```python
from build123d import *

# Parameters (mm, degrees)
SKETCH_1_R          = 9
EXTRUDE_1_DEPTH     = 65
SKETCH_2_R          = 6.5
SKETCH_2_R_2        = 5
CUT_EXTRUDE_1_DEPTH = 2
SKETCH_3_R          = 7.5
CUT_EXTRUDE_2_DEPTH = 0.25
CUT_EXTRUDE_START   = 1
SKETCH_4_R          = 6.75
SKETCH_4_R_2        = 5
CUT_EXTRUDE_3_DEPTH = 1
FILLET_1_R          = 1.5
FILLET_2_R          = 0.5
FILLET_3_R          = 0.5


with BuildPart() as part:
    # 草图1 → 凸台-拉伸1 (new body)
    with BuildSketch(Plane(origin=(0, 0, 0), x_dir=(1, 0, 0), z_dir=(0, 1, 0))):
        with Locations(Location((0, 0, 0), (0, 0, 270))):
            Circle(SKETCH_1_R)
    extrude(amount=EXTRUDE_1_DEPTH)

    # 草图2 → 切除-拉伸1 (cut)
    with BuildSketch(Plane(origin=(0, 65, 0), x_dir=(1, 0, 0), z_dir=(0, 1, 0))):
        with Locations(Location((0, 0, 0), (0, 0, 270))):
            Circle(SKETCH_2_R)
        with Locations(Location((0, 0, 0), (0, 0, 270))):
            Circle(SKETCH_2_R_2, mode=Mode.SUBTRACT)
    extrude(amount=-CUT_EXTRUDE_1_DEPTH, mode=Mode.SUBTRACT)

    # 草图3 → 切除-拉伸2 (cut)
    with BuildSketch(Plane(origin=(0, 0, 0), x_dir=(-1, 0, 0), z_dir=(0, -1, 0))):
        with Locations(Location((0, 0, 0), (0, 0, 90))):
            Circle(SKETCH_3_R)
    extrude(amount=-CUT_EXTRUDE_2_DEPTH, mode=Mode.SUBTRACT)

    # 草图4 → 切除-拉伸3 (cut)
    with BuildSketch(Plane(origin=(0, 63, 0), x_dir=(1, 0, 0), z_dir=(0, 1, 0)).offset(CUT_EXTRUDE_START)):
        with Locations(Location((0, 0, 0), (0, 0, 270))):
            Circle(SKETCH_4_R)
        with Locations(Location((0, 0, 0), (0, 0, 270))):
            Circle(SKETCH_4_R_2, mode=Mode.SUBTRACT)
    extrude(amount=-CUT_EXTRUDE_3_DEPTH, mode=Mode.SUBTRACT)

    # 圆角1
    fillet_1_edges = [part.edges().sort_by_distance(p)[0] for p in [
        (0, 0, -9),
        (0, 65, -9),
    ]]
    fillet(fillet_1_edges, radius=FILLET_1_R - 0.0001)  # a hair under: the kernel refuses the full size

    # 圆角2
    fillet_2_edges = [part.edges().sort_by_distance(p)[0] for p in [
        (0, 65, -6.5),
    ]]
    fillet(fillet_2_edges, radius=FILLET_2_R)

    # 圆角3
    fillet_3_edges = [part.edges().sort_by_distance(p)[0] for p in [
        (0, 63, -5),
        (0, 65, -5),
    ]]
    fillet(fillet_3_edges, radius=FILLET_3_R)


solid = part.part
```
The model under review builds one solid part; all positions refer to its coordinate system, in mm. A direction names the side the tool comes from. Coordinates: 2 decimals unless noted, no trailing zeros. Write each loop counter-clockwise with the first axis right and the second up, starting at its lowest first coordinate (ties: lowest second). Pieces come first, ordered by that corner, then holes. Notation, with made-up numbers: (74.5, 79) - (118.5, 79) arc R22 ccw to (118.5, 110) - close; hole circle Ø3 at (16.25, 55). An arc over 180 degrees is marked (long way). Answer in a Markdown table with one row per item. Add a question column.
Q1. Consider section A-A on y = 56. Give the boundary of the cut face in (x, z).
Q2. Clearance check with flat-ended pins moving along their axes: pin 1 (6 mm diameter, centred on x = -1.5, z = -1.5, fed in from -Y); pin 2 (8 mm diameter, centred on y = 9.5, z = -3.5, fed in from -X); pin 3 (3 mm diameter, centred on y = 55, z = -6.5, fed in from -X); pin 4 (8 mm diameter, centred on y = 54, z = -4.5, fed in from +X). State where each tip first meets the part, or that it passes through.
Q3. Draft analysis for pull direction Y (two halves, no side actions). For faces 1 (the face through (-7, 65, -2)), 2 (the face through (0, 63, -6)), 3 (the face through (0, 0.25, 0)), 4 (the face through (2.703, 32.066, 8.584)), state which applies: +Y half, -Y half, draft (parallel to the pull), parting line (faces both ways), or undercut.
Q4. To check wall thickness, follow line 1 along X through (y, z) = (63.45, 0); line 2 along X through (y, z) = (64.1, 0); line 3 along Y through (x, z) = (-0.75, -1.25). State the ranges of each line that lie inside material, in increasing order. Write a range as from..to.
Q5. For faces 5 (the face through (-3.955, 64.254, -5.158)), 6 (the face through (-6.59, 63.51, -1.46)), 7 (the face through (0, 65, 0)), list the 3-axis set-ups (+Z, -Z, +X, -X, +Y, -Y) from which the entire face can be reached by the end or side of a thin tool; tool diameter is ignored.
Answers below:
| question | item | result |
|---|---|---|
| 1 | outline | circle Ø18 at (0, 0) |
| 2 | pin 1 | y = 0.25 |
| 2 | pin 2 | x = -9 |
| 2 | pin 3 | x = -7.48 |
| 2 | pin 4 | x = 8.99 |
| 3 | face 1 | +Y half |
| 3 | face 2 | undercut |
| 3 | face 3 | -Y half |
| 3 | face 4 | draft |
| 4 | line 1 | -9..-6.75, -5..5, 6.75..9 |
| 4 | line 2 | -8.87..-6.5, -5..5, 6.5..8.87 |
| 4 | line 3 | 0.25..65 |
| 5 | face 5 | +Y |
| 5 | face 6 | none |
| 5 | face 7 | +Z, -Z, +X, -X, +Y |
